from build123d import *

# Parameters (mm, degrees)
F1_DEPTH  = 6.35
F2_SIZE   = 0.635
F1_FACE_R = 7.77875
F3_DEPTH  = 6.35
F4_R      = 5.08


with BuildPart() as f1:
    # F0 (on Front) → F1 (new body)
    with BuildSketch(Plane.XZ):
        with BuildLine():
            Line((25.4758205265, 31.9442898035), (25.4758205265, 39.7230398035))
            ThreePointArc((25.4758205265, 39.7230398035), (19.9754136523, 37.4446966777), (17.6970705265, 31.9442898035))
            Line((17.6970705265, 31.9442898035), (25.4758205265, 31.9442898035))
        make_face()
        with BuildLine():
            Line((25.4758205265, 31.9442898035), (33.2545705265, 31.9442898035))
            ThreePointArc((33.2545705265, 31.9442898035), (30.9762274006, 37.4446966777), (25.4758205265, 39.7230398035))
            Line((25.4758205265, 39.7230398035), (25.4758205265, 31.9442898035))
        make_face()
        with BuildLine():
            ThreePointArc((25.4758205265, 24.1655398035), (30.9762274006, 26.4438829294), (33.2545705265, 31.9442898035))
            Line((33.2545705265, 31.9442898035), (25.4758205265, 31.9442898035))
            Line((25.4758205265, 31.9442898035), (25.4758205265, 24.1655398035))
        make_face()
        with BuildLine():
            ThreePointArc((17.6970705265, 31.9442898035), (19.9754136523, 26.4438829294), (25.4758205265, 24.1655398035))
            Line((25.4758205265, 24.1655398035), (25.4758205265, 31.9442898035))
            Line((25.4758205265, 31.9442898035), (17.6970705265, 31.9442898035))
        make_face()
    extrude(amount=-F1_DEPTH)

    # F2
    f2_edges = [f1.edges().sort_by_distance(p)[0] for p in [
        (33.254571, 6.35, 31.94429),
    ]]
    chamfer(f2_edges, length=F2_SIZE)

    # F0 (on Front) + F1_face (on face) → F3 (join)
    with BuildSketch(Plane.XZ):
        with BuildLine():
            ThreePointArc((25.4758205265, 39.7230398035), (30.9762274006, 37.4446966777), (33.2545705265, 31.9442898035))
            Line((33.2545705265, 31.9442898035), (36.9058205265, 31.9442898035))
            ThreePointArc((36.9058205265, 31.9442898035), (25.4758205265, 43.3742898035), (14.0458205265, 31.9442898035))
            Line((14.0458205265, 31.9442898035), (17.6970705265, 31.9442898035))
            ThreePointArc((17.6970705265, 31.9442898035), (19.9754136523, 37.4446966777), (25.4758205265, 39.7230398035))
        make_face()
        with BuildLine():
            Line((36.9058205265, 31.9442898035), (33.2545705265, 31.9442898035))
            ThreePointArc((33.2545705265, 31.9442898035), (30.9762274006, 26.4438829294), (25.4758205265, 24.1655398035))
            ThreePointArc((25.4758205265, 24.1655398035), (19.9754136523, 26.4438829294), (17.6970705265, 31.9442898035))
            Line((17.6970705265, 31.9442898035), (14.0458205265, 31.9442898035))
            ThreePointArc((14.0458205265, 31.9442898035), (25.4758205265, 20.5142898035), (36.9058205265, 31.9442898035))
        make_face()
    with BuildSketch(Plane(origin=(25.4758205265, 0, 31.9442898035), x_dir=(1, 0, 0), z_dir=(0, -1, 0))):
        Circle(F1_FACE_R)
    extrude(amount=F3_DEPTH)

    # F4
    f4_edges = [f1.edges().sort_by_distance(p)[0] for p in [
        (36.905821, -6.35, 31.94429),
    ]]
    fillet(f4_edges, radius=F4_R)


solid = f1.part
Input: part model. Units: mm. Frame: model coordinates. A direction names the side the tool comes from. Give positions to 0.01 mm unless a question says otherwise; leave off trailing zeros. Write each loop counter-clockwise with the first axis right and the second up, starting at its lowest first coordinate (ties: lowest second). Pieces come first, ordered by that corner, then holes.
Q1. Section B-B, the plane y = -3.5. Output: boundary loops of the cut face in (x, z), plus the area to 3 significant figures.
Q2. First-contact query: P1, Ø1, axis at x = 19, z = 36.5, coming from the +Y side; P2, Ø1, axis at y = 4.5, z = 35, coming from the -X side; P3, Ø6, axis at y = 0.5, z = 38, coming from the -X side. Flat tips, straight axial feed; report the tip coordinate or a pass-through.
Q3. Material intervals for probe 1 along Z at (x, y) = (21, -1); probe 2 along X at (y, z) = (0.5, 28.25); probe 3 along X at (y, z) = (-4.75, 35.25), sorted ascending.
Q4. Section C-C, the plane y = -2. Output: boundary loops of the cut face in (x, z), plus the area to 3 significant figures.
Q5. Set-up query: faces 1 (the face through (28, 0, 24)), 2 (the face through (25, -6.35, 32)). Return all of +Z, -Z, +X, -X, +Y, -Y with unobstructed straight access to the full face (end or side cutting, diameter ignored); none if empty.
Q6. Section A-A, the plane y = 2.75. Output: boundary loops of the cut face in (x, z).
Filled in:
1. outline: circle Ø21.83 at (25.48, 31.94)
1. area: 374 mm2
2. P1: stops at y = 6.08
2. P2: stops at x = 18.13
2. P3: stops at x = 14.47
3. probe 1: z = 21.43 to 42.46
3. probe 2: x = 18.63 to 32.32
3. probe 3: x = 15.98 to 34.97
4. outline: circle Ø22.75 at (25.48, 31.94)
4. area: 407 mm2
5. face 1: +Y
5. face 2: +Z, -Z, +X, -X, -Y
6. outline: circle Ø15.56 at (25.48, 31.94)
